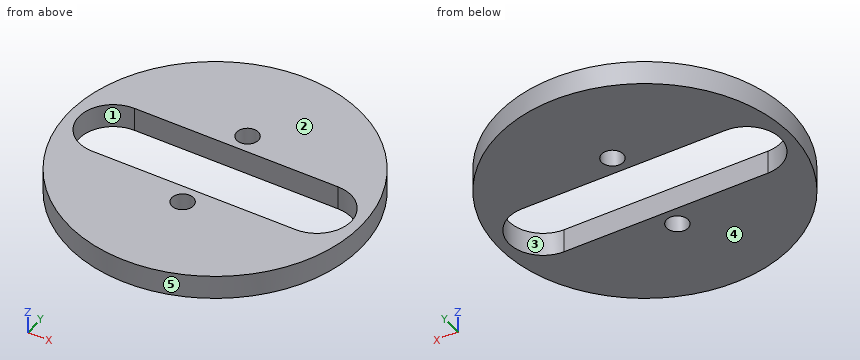
Autodesk Inventor part; units mm, degrees
ref_plane "YZ Plane" through (0, 0, 0) normal (1, 0, 0) x (0, 1, 0)
ref_plane "XZ Plane" through (0, 0, 0) normal (0, 1, 0) x (-1, 0, 0)
ref_plane "XY Plane" through (0, 0, 0) normal (0, 0, 1) x (1, 0, 0)
sketch "Sketch1" plane through (0, 0, 0) normal (0, 0, 1) x (1, 0, 0)
  circle A0 centre (0, 0) radius 22
  dimension "d0" = 44
extrude "Extrusion1" add sketch "Sketch1" along normal blind 3.6
sketch "Sketch2" plane through (0, 0, 3.6) normal (0, 0, 1) x (1, 0, 0)
  line L0 (15.3, 0) -> (-15.3, 0) construction
  line L1 (15.3, 5.15) -> (-15.3, 5.15)
  line L2 (-15.3, -5.15) -> (15.3, -5.15)
  arc A0 (15.3, -5.15) -> (15.3, 5.15) centre (15.3, 0) ccw
  arc A1 (-15.3, 5.15) -> (-15.3, -5.15) centre (-15.3, 0) ccw
  point P0 (0, 0)
  dimension "d3" = 15.3
  dimension "d4" = 10.3
extrude "Extrusion2" cut sketch "Sketch2" against normal blind 3.6
sketch "Sketch3" plane through (0, 0, 3.6) normal (0, 0, 1) x (1, 0, 0)
  line L0 (-2.6, 9.8) -> (2.6, 9.8)
  line L1 (2.6, 9.8) -> (2.6, 6)
  line L2 (2.6, 6) -> (-2.6, 6)
  line L3 (-2.6, 6) -> (-2.6, 9.8)
  line L4 (-2.6, 9.8) -> (2.6, 6) construction
  line L5 (2.6, 9.8) -> (-2.6, 6) construction
  line L6 (-30.8, 0) -> (30.8, 0)
  line L7 (-30.8, 0) -> (30.8, 0)
  line L8 (-2.6, -9.8) -> (2.6, -9.8)
  line L9 (2.6, -9.8) -> (2.6, -6)
  line L10 (2.6, -6) -> (-2.6, -6)
  line L11 (-2.6, -6) -> (-2.6, -9.8)
  line L12 (-2.6, -9.8) -> (2.6, -6) construction
  line L13 (2.6, -9.8) -> (-2.6, -6) construction
  circle A0 centre (0, -7.9) radius 1.625
  circle A1 centre (0, 7.9) radius 1.625
  point P0 (0, 0)
  dimension "d7" = 5.2
  dimension "d8" = 3.8
  dimension "d9" = 6
  dimension "d10" = 6
  dimension "d13" = 0
  dimension "d14" = 3.25
  dimension "d15" = 3.25
extrude "Extrusion3" cut sketch "Sketch3" against normal blind 10 contours A0 | A1
properties part number "1"
The listing builds one solid part. Answer for the finished solid, in the listing's coordinates (mm). Face numbers are marked on the shaded views. A direction names the side the tool comes from. Coordinates: 2 decimals unless noted, no trailing zeros. Order: outer loops, then holes, each group sorted by start corner. A loop starts at its lowest first (then second) coordinate and runs counter-clockwise, first axis right, second up.
Q1. A cutting plane is placed at D-D, the plane x = -0.5. Write down the section's boundary in (y, z).
Q2. For a pull along X with two mould halves and no side action, classify the marked faces 3, 4 and 5 as pulls with the +X half, pulls with the -X half, needs draft (parallel to the pull), parting line crosses it, or undercut.
Q3. Which of the six approach directions +Z, -Z, +X, -X, +Y, -Y give full straight-line access (tool end or side, diameter ignored) to the marked faces 1 and 2?
Q4. Consider line 1 (Y direction, x = 0, z = 2.4) (3 decimals); line 2 (Y direction, x = 0.5, z = 0.25); line 3 (Y direction, x = -8, z = 1.65). Determine where each line is inside the solid, lowest interval first.
Q5. Given P1, Ø1.9, axis at x = 0, y = 7.9, coming from the -Z side; P2, Ø1.5, axis at x = -14.5, y = 10.5, coming from the -Z side; P3, Ø1.8, axis at x = 6, z = 1.5, coming from the +Y side; P4, Ø1.8, axis at x = -2.5, z = 1.5, coming from the -Y side, each flat-ended and moving along its own axis, determine where each tip first touches the part or whether it passes through.
Q6. A cutting plane is placed at A-A, the plane z = 1.25. Write down the section's boundary in (x, y) (3 decimals), and give its area (3 significant figures).
Q7. A cutting plane is placed at C-C, the plane x = -11. Write down the section's boundary in (y, z), and give its area (3 significant figures).
Q8. A cutting plane is placed at B-B, the plane y = 0. Write down the section's boundary in (x, z), and give its area (3 significant figures).
Answers follow:
1. outline: (-21.99, 0) - (-9.45, 0) - (-9.45, 3.6) - (-21.99, 3.6) - close; (-6.35, 0) - (-5.15, 0) - (-5.15, 3.6) - (-6.35, 3.6) - close; (5.15, 0) - (6.35, 0) - (6.35, 3.6) - (5.15, 3.6) - close; (9.45, 0) - (21.99, 0) - (21.99, 3.6) - (9.45, 3.6) - close
2. face 3: undercut
2. face 4: needs draft
2. face 5: parting line crosses it
3. face 1: +Z, -Z
3. face 2: +Z, +X, -X, +Y, -Y
4. line 1: y = -22 to -9.525, -6.275 to -5.15, 5.15 to 6.275, 9.525 to 22
4. line 2: y = -21.99 to -9.45, -6.35 to -5.15, 5.15 to 6.35, 9.45 to 21.99
4. line 3: y = -20.49 to -5.15, 5.15 to 20.49
5. P1: passes through
5. P2: stops at z = 0
5. P3: stops at y = 21.4
5. P4: stops at y = -21.94
6. outline: circle Ø44 at (0, 0); hole (-15.3, -5.15) - (15.3, -5.15) arc R5.15 ccw to (15.3, 5.15) - (-15.3, 5.15) arc R5.15 ccw to start; hole circle Ø3.25 at (0, -7.9); hole circle Ø3.25 at (0, 7.9)
6. area: 1,110 mm2
7. outline: (-19.05, 0) - (-5.15, 0) - (-5.15, 3.6) - (-19.05, 3.6) - close; (5.15, 0) - (19.05, 0) - (19.05, 3.6) - (5.15, 3.6) - close
7. area: 100 mm2
8. outline: (-22, 0) - (-20.45, 0) - (-20.45, 3.6) - (-22, 3.6) - close; (20.45, 0) - (22, 0) - (22, 3.6) - (20.45, 3.6) - close
8. area: 11.2 mm2
